Answer from the drawing. Dimensions are ordinates in mm from the lowest x, y and z of the part. Give positions to 0.01 mm unless a question says otherwise; leave off trailing zeros. Write each loop counter-clockwise with the first axis right and the second up, starting at its lowest first coordinate (ties: lowest second). Pieces come first, ordered by that corner, then holes. Notation, with made-up numbers: (-7.5, 4) -> (22.5, 4) arc R13 cw to (22.5, 23) -> close; hole circle Ø6 at (-9, 52.5). An arc over 180 degrees is marked (long way). Use a Markdown table: item, result. Add a question column.
Q1. Section A-A, the plane x = 69.85 is taken. Give the vertices of the cut face in (y, z).
Q2. Section D-D, the plane z = 93 is taken. Give the vertices of the cut face in (x, y), plus the area to 3 significant figures.
Q3. Consider line 1 (Z direction, x = 36.5, y = 19.5); line 2 (X direction, y = 49, z = 88); line 3 (Y direction, x = 71.5, z = 37). Determine where each line is inside the solid, lowest interval first.
Q4. Section C-C, the plane y = 50.8 is taken. Give the vertices of the cut face in (x, z), plus the area to 3 significant figures.
Q5. For a pull along Z with two mould halves and no side action, classify the marked faces 1, 2 and 3 as pulls with the +Z half, pulls with the -Z half, needs draft (parallel to the pull), parting line crosses it, or undercut.
Q6. Each of these flat-tipped pins is pushed along its axis until it touches: pin 1 Ø1 at (y, z) = (62.5, 30.5) entering from +X; pin 2 Ø1.5 at (x, z) = (64, 80) entering from -Y; pin 3 Ø3 at (x, y) = (118, 80) entering from +Z. Where does it stop, or does it pass through?
Q7. Section B-B, the plane y = 28 is taken. Give the vertices of the cut face in (x, z).
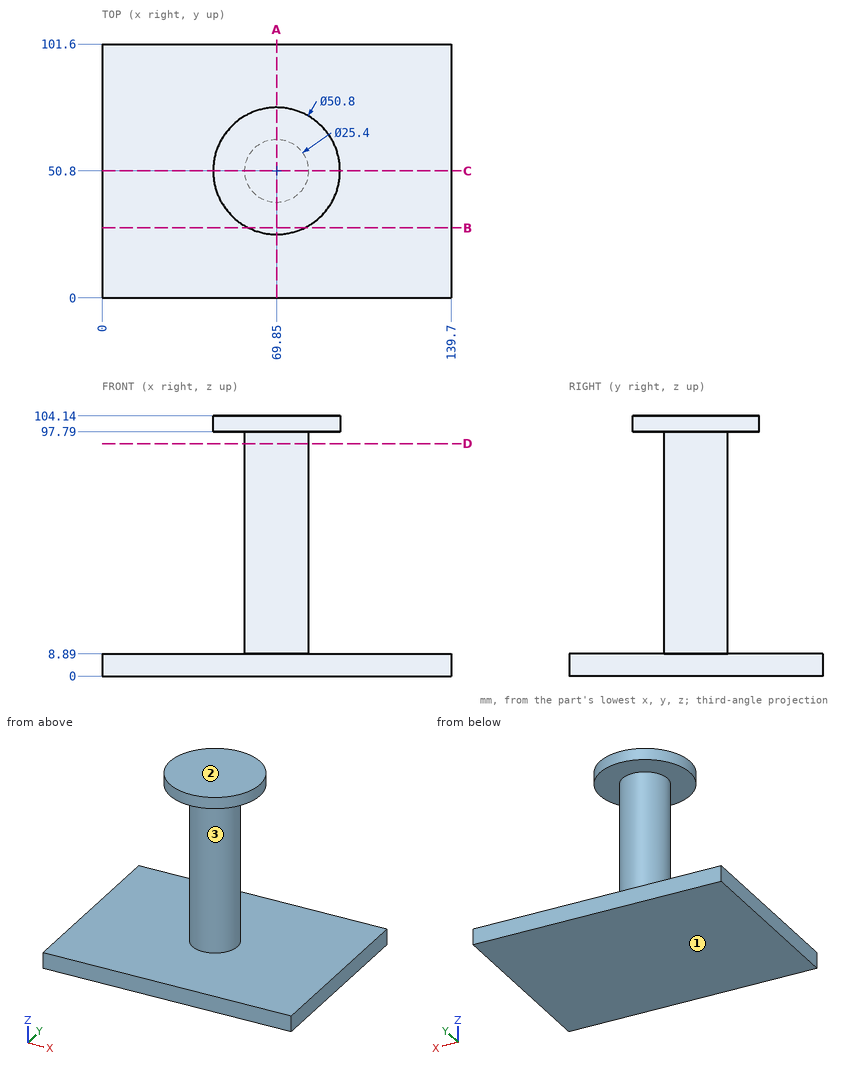
Result set:
| question | item | result |
|---|---|---|
| 1 | outline | (0, 0) -> (101.6, 0) -> (101.6, 8.89) -> (63.5, 8.89) -> (63.5, 97.79) -> (76.2, 97.79) -> (76.2, 104.14) -> (25.4, 104.14) -> (25.4, 97.79) -> (38.1, 97.79) -> (38.1, 8.89) -> (0, 8.89) -> close |
| 2 | outline | circle Ø25.4 at (69.85, 50.8) |
| 2 | area | 507 mm2 |
| 3 | line 1 | z = 0 to 8.89 |
| 3 | line 2 | x = 57.28 to 82.42 |
| 3 | line 3 | y = 38.21 to 63.39 |
| 4 | outline | (0, 0) -> (139.7, 0) -> (139.7, 8.89) -> (82.55, 8.89) -> (82.55, 97.79) -> (95.25, 97.79) -> (95.25, 104.14) -> (44.45, 104.14) -> (44.45, 97.79) -> (57.15, 97.79) -> (57.15, 8.89) -> (0, 8.89) -> close |
| 4 | area | 3,820 mm2 |
| 5 | face 1 | pulls with the -Z half |
| 5 | face 2 | pulls with the +Z half |
| 5 | face 3 | undercut |
| 6 | pin 1 | stops at x = 75.84 |
| 6 | pin 2 | stops at y = 39.17 |
| 6 | pin 3 | stops at z = 8.89 |
| 7 | outline | (0, 0) -> (139.7, 0) -> (139.7, 8.89) -> (0, 8.89) -> close; (58.66, 97.79) -> (81.04, 97.79) -> (81.04, 104.14) -> (58.66, 104.14) -> close |
